from build123d import *

# Parameters (mm, degrees)
SKETCH2_W                 = 19.05
SKETCH2_H                 = 76.2
BOSS_EXTRUDE2_DEPTH       = 0.508
EDGE_FLANGE2_DEPTH        = 76.2
F_4_CLEARANCE_HOLE1_D     = 3.2639
F_4_CLEARANCE_HOLE1_DEPTH = 0.508


# Sheet-metal steps are written as plain solids
with BuildPart() as part:
    # Sketch2 → Boss-Extrude2 (new body)
    with BuildSketch(Plane(origin=(0, 0, 0), x_dir=(1, 0, 0), z_dir=(0, 1, 0))):
        with Locations((-9.525, 38.1)):
            Rectangle(SKETCH2_W, SKETCH2_H)
    extrude(amount=BOSS_EXTRUDE2_DEPTH)

    # Edge-Flange2 section (across the edge) → Edge-Flange2 (add)
    with BuildSketch(Plane(origin=(7.665128061, 0.508, 0), x_dir=(-0.7071067811865488, -0.7071067811865464, 0), z_dir=(0, 0, -1))):
        with BuildLine():
            Line((-0.508, 7.665128061), (-0.508, 57.15))
            Line((-0.508, 57.15), (0, 57.15))
            Line((0, 57.15), (0, 7.665128061))
            ThreePointArc((0, 7.665128061), (1.959980102, 4.731810545), (5.42006403, 5.42006403))
            Line((5.42006403, 5.42006403), (5.779274275, 5.060853785))
            ThreePointArc((5.779274275, 5.060853785), (1.765576919, 4.262479742), (-0.508, 7.665128061))
        make_face()
    extrude(amount=EDGE_FLANGE2_DEPTH)

    # #4 Clearance Hole1
    with Locations(Plane(origin=(0, 0, 0), x_dir=(-1, 0, 0), z_dir=(0, -1, 0))):
        with Locations((9.525, 69.85), (9.525, 6.35)):
            Hole(F_4_CLEARANCE_HOLE1_D / 2, depth=F_4_CLEARANCE_HOLE1_DEPTH)


solid = part.part
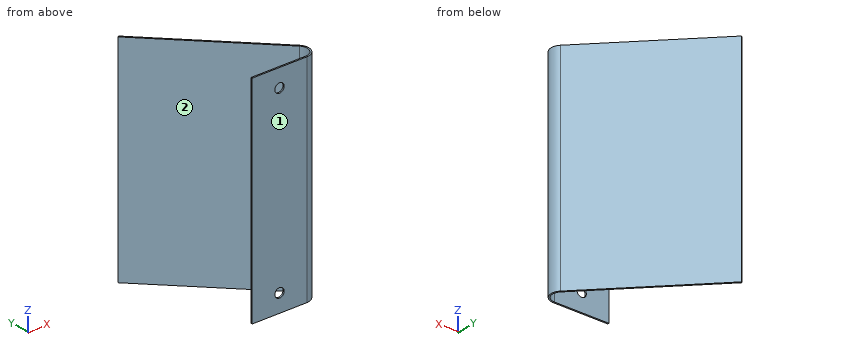
The listing builds one solid part. Answer for the finished solid, in the listing's coordinates (mm). Face numbers are marked on the shaded views. A direction names the side the tool comes from. Round coordinates to 2 decimals unless told otherwise and drop trailing zeros. Write each loop counter-clockwise with the first axis right and the second up, starting at its lowest first coordinate (ties: lowest second). Pieces come first, ordered by that corner, then holes. Notation, with made-up numbers: (47.25, 87.5) - (59.25, 87.5) arc R25 cw to (59.25, 106.5) - close; hole circle Ø3 at (21, -37.75). An arc over 180 degrees is marked (long way). Use one line per item in the form item = value. Start each with the question number.
Item 1: Find the intervals of material crossed by line 1 (Y direction, x = -1.5, z = -71.5); line 2 (Y direction, x = -1, z = -15); line 3 (X direction, y = 11, z = -10), in increasing order. Write a range as [from, to].
Item 2: A cutting plane is placed at B-B (x = -9.5). Write down the section's boundary in (y, z).
Item 3: Flat-ended cylindrical pins translate along their axes: pin 1 Ø6 at (x, z) = (-26.5, -26.5) entering from -Y; pin 2 Ø3 at (x, z) = (-9.525, -69.85) entering from +Y; pin 3 Ø8 at (y, z) = (34.5, -10.5) entering from -X. Find the tip coordinate at first contact, or state that the pin passes through.
Item 4: A tool of negligible diameter and unlimited length cuts with its end or side. For the marked faces 1 and 2, from which of +Z, -Z, +X, -X, +Y, -Y can it reach the whole face along a straight path? Write none if from no direction.
Item 5: A cutting plane is placed at D-D (x = -26). Write down the section's boundary in (y, z), plus the area to 3 significant figures.
Item 6: A cutting plane is placed at C-C (z = -36). Write down the section's boundary in (x, y) (3 decimals), plus the area to 3 significant figures.
Item 7: A cutting plane is placed at A-A (z = -69.85). Write down the section's boundary in (x, y) (3 decimals).
The answers:
q1.line_1 = [0, 0.51], [9.67, 10.39]
q1.line_2 = [0, 0.51], [9.17, 9.89]
q1.line_3 = [-2.83, -2.11]
q2.outline = (0, -76.2) - (0.51, -76.2) - (0.51, -71.48) - (0, -71.48) - close; (0, -68.22) - (0.51, -68.22) - (0.51, -7.98) - (0, -7.98) - close; (0, -4.72) - (0.51, -4.72) - (0.51, 0) - (0, 0) - close; (17.67, -76.2) - (18.39, -76.2) - (18.39, 0) - (17.67, 0) - close
q3.pin_1 = 31.67
q3.pin_2 = 19.92
q3.pin_3 = -30.33
q4.face_1 = +Z, -Z, +X, -X, -Y
q4.face_2 = +Z, -Z, -X
q5.outline = (34.17, -76.2) - (34.89, -76.2) - (34.89, 0) - (34.17, 0) - close
q5.area = 54.7 mm^2
q6.outline = (-32.746, 40.919) - (2.245, 5.928) arc R3.175 cw to (0, 0.508) - (-19.05, 0.508) - (-19.05, 0) - (0, 0) arc R3.683 ccw to (2.604, 6.287) - (-32.387, 41.278) - close
q6.area = 38.9 mm^2
q7.outline = (-32.746, 40.919) - (2.245, 5.928) arc R3.175 cw to (0, 0.508) - (-7.893, 0.508) - (-7.893, 0) - (0, 0) arc R3.683 ccw to (2.604, 6.287) - (-32.387, 41.278) - close; (-19.05, 0) - (-11.157, 0) - (-11.157, 0.508) - (-19.05, 0.508) - close
